Study the drawing (mm; zero at the part's minimum x, y, z) and answer. Give positions to 0.01 mm unless a question says otherwise; leave off trailing zeros. Write each loop counter-clockwise with the first axis right and the second up, starting at its lowest first coordinate (ties: lowest second). Pieces come first, ordered by that corner, then holes. Notation, with made-up numbers: (-6.5, 83) - (31.5, 83) arc R21 ccw to (31.5, 95) - close; hole circle Ø1 at (-27, 63.25). An arc over 180 degrees is marked (long way). Return JSON: item names as keys, results as strings.
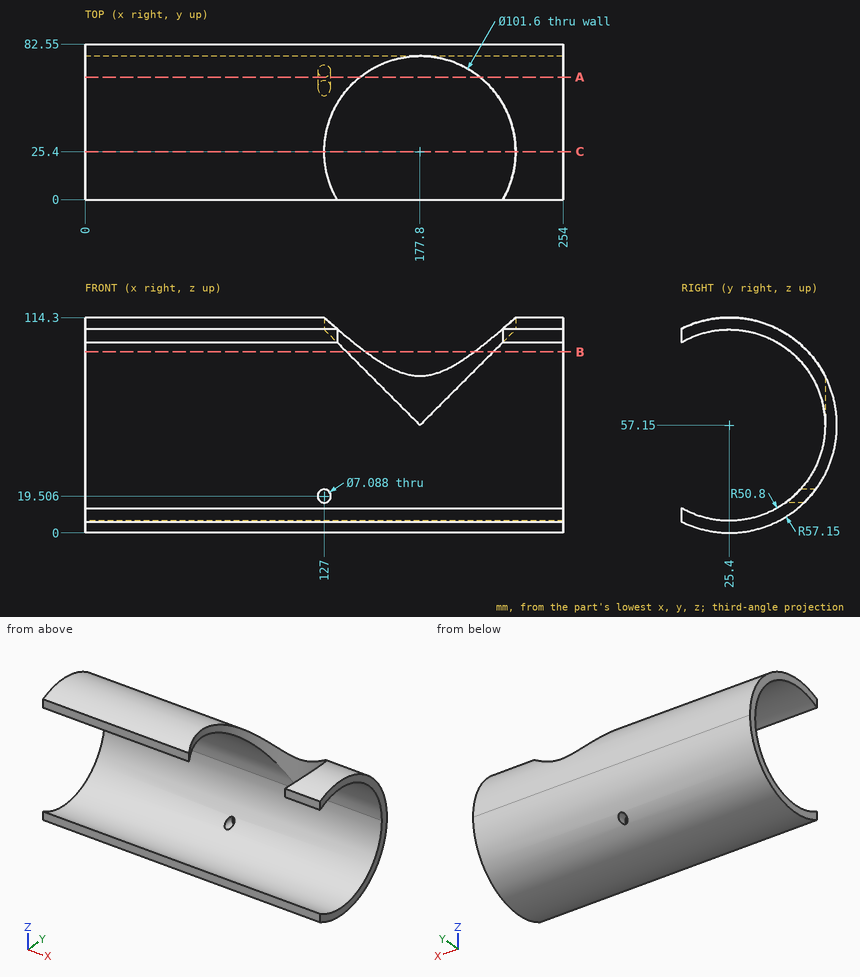
Item 1: A cutting plane is placed at C-C on y = 25.4. Determine the outline of the cut face in (x, z), then the cut area to 3 significant figures.
Answer below:
{"outline": "(0, 0) - (254, 0) - (254, 6.35) - (0, 6.35) - close; (0, 107.95) - (127, 107.95) - (127, 114.3) - (0, 114.3) - close; (228.6, 107.95) - (254, 107.95) - (254, 114.3) - (228.6, 114.3) - close", "area": "2,580 mm²"}
Item 2: Flat-ended cylindrical pins translate along their axes: P1, Ø4, axis at x = 69.5, z = 99, coming from the -Y side; P2, Ø8, axis at x = 39, y = 32, coming from the +Z side; P3, Ø2, axis at x = 73, z = 38, coming from the +Y side. Find the tip coordinate at first contact, or state that the pin passes through.
Answer below:
{"P1": "stops at y = 51.05", "P2": "stops at z = 114.24", "P3": "stops at y = 79.59"}
Item 3: A cutting plane is placed at B-B on z = 96. Determine the outline of the cut face in (x, y), then the cut area to 3 significant figures.
Answer below:
{"outline": "(0, 58.13) - (138.95, 58.13) arc R50.8 cw to (149.1, 67.31) - (0, 67.31) - close; (206.5, 67.31) arc R50.8 cw to (216.65, 58.13) - (254, 58.13) - (254, 67.31) - close", "area": "1,700 mm²"}
Item 4: A cutting plane is placed at A-A on y = 65. Determine the outline of the cut face in (x, z), then the cut area to 3 significant figures.
Answer below:
{"outline": "(0, 15.94) - (254, 15.94) - (254, 25.33) - (0, 25.33) - close; (0, 88.97) - (145.98, 88.97) - (145.98, 98.36) - (0, 98.36) - close; (209.62, 88.97) - (254, 88.97) - (254, 98.36) - (209.62, 98.36) - close; hole circle Ø7.09 at (127, 19.51)", "area": "4,130 mm²"}
Item 5: Consider L1, parallel to Z at x = 244.5, y = 57.5 (1 decimal); L2, parallel to Z at x = 14, y = 65 (1 decimal); L3, parallel to Z at x = 227.5, y = 23. Determine where each line is inside the solid, lowest interval first.
Answer below:
{"L1": "z = 9.9 to 17.8, 96.5 to 104.4", "L2": "z = 15.9 to 25.3, 89 to 98.4", "L3": "z = 0.05 to 6.41"}
